Drawing for the job (mm, zero at the part's lowest x, y, z). A direction names the side the tool comes from. Give positions to 0.01 mm unless a question says otherwise; leave off trailing zeros. Order: outer loops, then holes, each group sorted by start corner. A loop starts at its lowest first (then second) coordinate and runs counter-clockwise, first axis right, second up. Notation, with made-up numbers: M 32.5,41 L 71.5,41 A13 cw 71.5,51 Z; hole C -40,-39 d11. An arc over 180 degrees is marked long. One line per item, written item: value.
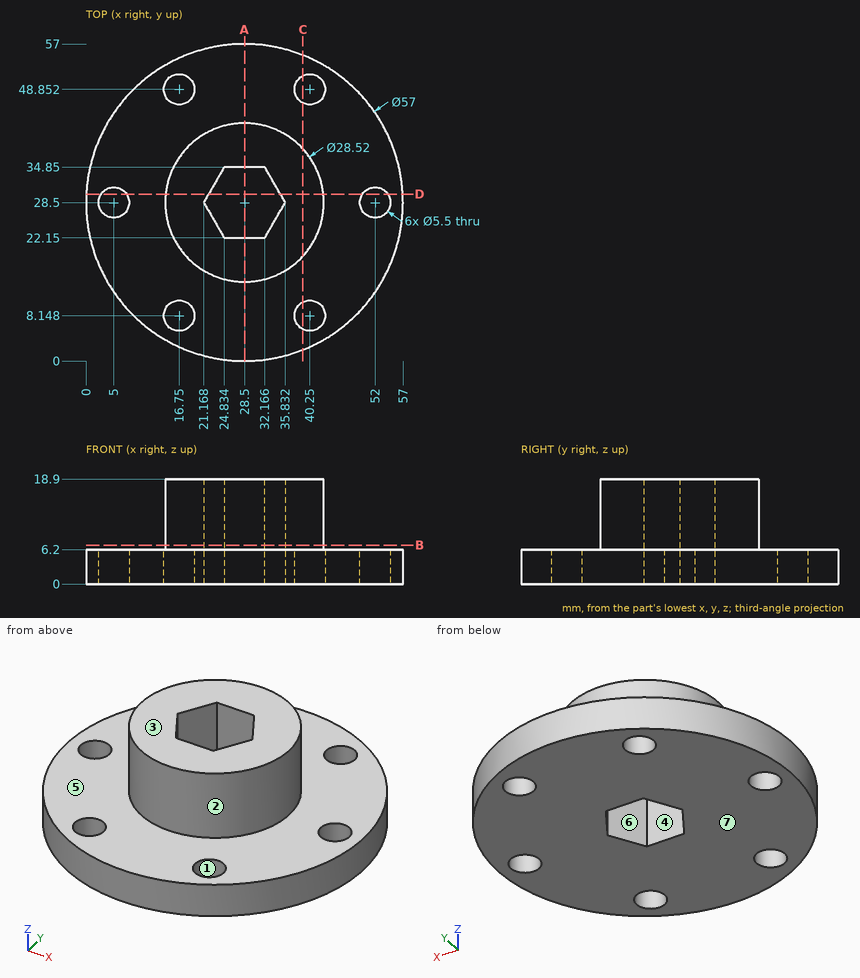
1) Drill centre lines: probe 1 along X at (y, z) = (6, 5) (1 decimal); probe 2 along Y at (x, z) = (40.25, 2) (1 decimal); probe 3 along Y at (x, z) = (34.5, 7.5) (1 decimal). Where is each one in solid material? Low to high. Write a range as from..to.
Check values:
probe 1: 11..15, 18.5..38.5, 42..46
probe 2: 2.5..5.4, 10.9..46.1, 51.6..54.5
probe 3: 15.6..26.2, 30.8..41.4
2) Pin check, flat tips, straight feed: pin 1 (3 mm diameter, centred on x = 19, z = 6.5, fed in from -Y) (1 decimal); pin 2 (6 mm diameter, centred on x = 29.5, y = 49, fed in from -Z); pin 3 (3.5 mm diameter, centred on x = 27.5, z = 10, fed in from -Y); pin 4 (2 mm diameter, centred on y = 9, z = 2, fed in from +X). Stop position of each tip, or through.
Check values:
pin 1: y = 1.2
pin 2: z = 0
pin 3: y = 14.24
pin 4: x = 50.18
3) Saw through at B-B, the plane z = 7. Write the cut outline in (x, y).
Check values:
outline: C 28.5,28.5 d28.52; hole M 21.17,28.5 L 24.83,22.15 L 32.17,22.15 L 35.83,28.5 L 32.17,34.85 L 24.83,34.85 Z
4) Saw through at C-C, the plane x = 39. Write the cut outline in (y, z) (1 decimal), then the cut area to 3 significant figures.
Check values:
outline: M 2,0 L 5.7,0 L 5.7,6.2 L 2,6.2 Z; M 10.6,0 L 46.4,0 L 46.4,6.2 L 38.1,6.2 L 38.1,18.9 L 18.9,18.9 L 18.9,6.2 L 10.6,6.2 Z; M 51.3,0 L 55,0 L 55,6.2 L 51.3,6.2 Z
area: 513 mm^2
5) Saw through at D-D, the plane y = 30. Write the cut outline in (x, z) (1 decimal).
Check values:
outline: M 0,0 L 2.7,0 L 2.7,6.2 L 0,6.2 Z; M 7.3,0 L 22,0 L 22,18.9 L 14.3,18.9 L 14.3,6.2 L 7.3,6.2 Z; M 35,0 L 49.7,0 L 49.7,6.2 L 42.7,6.2 L 42.7,18.9 L 35,18.9 Z; M 54.3,0 L 57,0 L 57,6.2 L 54.3,6.2 Z
6) Saw through at A-A, the plane x = 28.5. Write the cut outline in (y, z).
Check values:
outline: M 0,0 L 22.15,0 L 22.15,18.9 L 14.24,18.9 L 14.24,6.2 L 0,6.2 Z; M 34.85,0 L 57,0 L 57,6.2 L 42.76,6.2 L 42.76,18.9 L 34.85,18.9 Z
7) Tool access for the marked faces 5, 6 and 7: list every direction of +Z, -Z, +X, -X, +Y, -Y with a clear straight run to the whole face (end or side of a thin tool).
Check values:
face 5: +Z
face 6: +Z, -Z
face 7: -Z, +X, -X, +Y, -Y
8) Mould opens along Y. For the marked faces 1, 2, 3 and 4 say: released by +Y, released by -Y, zero draft, split by the parting line, or undercut.
Check values:
face 1: undercut
face 2: split by the parting line
face 3: zero draft
face 4: undercut
